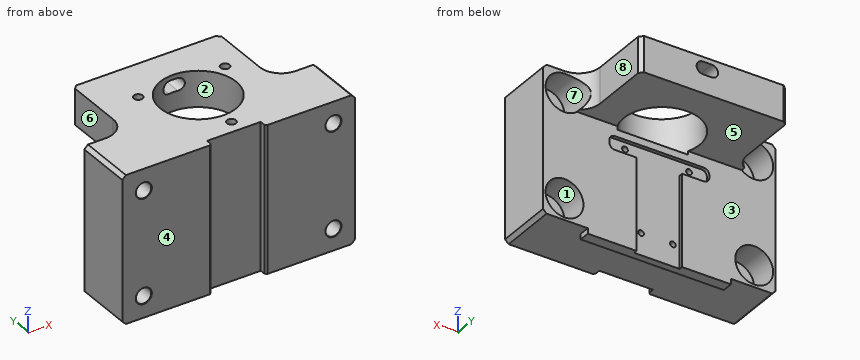
from build123d import *

# Parameters (mm, degrees)
SKETCH1_W                                     = 65
SKETCH1_H                                     = 41
BOSS_EXTRUDE1_DEPTH                           = 16
SKETCH15_W                                    = 41
SKETCH15_H                                    = 10
BOSS_EXTRUDE4_DEPTH                           = 23
SKETCH4_R                                     = 10.6
CUT_EXTRUDE3_DEPTH                            = 11
M3_TAPPED_HOLE1_D                             = 2.5
M3_TAPPED_HOLE1_DEPTH                         = 8.5
M3_TAPPED_HOLE1_TIP                           = 0.751075774
CUT_EXTRUDE4_START                            = -1
CUT_EXTRUDE4_DEPTH                            = 1
SKETCH30_W                                    = 40
SKETCH30_H                                    = 3
BOSS_EXTRUDE5_DEPTH                           = 1.5
SKETCH27_W                                    = 12.7
SKETCH27_H                                    = 4.1
CUT_EXTRUDE6_DEPTH                            = 1
CUT_EXTRUDE7_DEPTH                            = 1
M2_TAPPED_HOLE1_D                             = 1.6
M2_TAPPED_HOLE1_DEPTH                         = 6
M2_TAPPED_HOLE1_TIP                           = 0.480688495
CBORE_FOR_M4_HEX_HEAD_MACHINE_SCREW1_AT_COUNT = 2
CBORE_FOR_M4_HEX_HEAD_MACHINE_SCREW1_AT_PITCH = 53
CBORE_FOR_M4_HEX_HEAD_MACHINE_SCREW1_2_COUNT  = 2
CBORE_FOR_M4_HEX_HEAD_MACHINE_SCREW1_2_PITCH  = 60.415229868
CBORE_FOR_M4_HEX_HEAD_MACHINE_SCREW1_3_COUNT  = 2
CBORE_FOR_M4_HEX_HEAD_MACHINE_SCREW1_3_PITCH  = 29
CHAMFER4_SIZE                                 = 1
F_3_5_START                                   = 44
F_3_5_3_5_DIAMETER_SLOT1_DEPTH                = 10
FILLET1_R                                     = 6
SKETCH33_W                                    = 15
SKETCH33_H                                    = 41
CUT_EXTRUDE8_DEPTH                            = 2
CHAMFER5_SIZE                                 = 0.5


with BuildPart() as part:
    # Sketch1 → Boss-Extrude1 (new body)
    with BuildSketch(Plane(origin=(0, 15, 0), x_dir=(1, 0, 0), z_dir=(0, 1, 0))):
        with Locations((0, 20)):
            Rectangle(SKETCH1_W, SKETCH1_H)
    extrude(amount=BOSS_EXTRUDE1_DEPTH)

    # Sketch15 → Boss-Extrude4 (add)
    with BuildSketch(Plane(origin=(0, 31, 0), x_dir=(1, 0, 0), z_dir=(0, 1, 0))):
        with Locations((0, 4.5)):
            Rectangle(SKETCH15_W, SKETCH15_H)
    extrude(amount=BOSS_EXTRUDE4_DEPTH)

    # Sketch4 → Cut-Extrude3 (cut)
    with BuildSketch(Plane.XY.offset(0.5)):
        with Locations((1.85, 34.8)):
            Circle(SKETCH4_R)
    extrude(amount=-CUT_EXTRUDE3_DEPTH, mode=Mode.SUBTRACT)

    # M3 Tapped Hole1
    with Locations(Plane.XY.offset(0.5)):
        with Locations((13.974355653, 41.8), (1.85, 20.8), (-10.274355653, 41.8)):
            Hole(M3_TAPPED_HOLE1_D / 2, depth=M3_TAPPED_HOLE1_DEPTH)
            with Locations((0, 0, -(M3_TAPPED_HOLE1_DEPTH + M3_TAPPED_HOLE1_TIP / 2))):  # 118° drill point
                Cone(0, M3_TAPPED_HOLE1_D / 2, M3_TAPPED_HOLE1_TIP, mode=Mode.SUBTRACT)

    # Sketch16 → Cut-Extrude4 (cut)
    with BuildSketch(Plane(origin=(0, 31, 0), x_dir=(1, 0, 0), z_dir=(0, 1, 0)).offset(CUT_EXTRUDE4_START)):
        Polygon((-10.95, 12.5), (10.95, 12.5), (10.95, 16.3), (6.35, 16.3), (6.35, 37.9), (-6.35, 37.9), (-6.35, 16.3), (-10.95, 16.3), align=None)
    extrude(amount=CUT_EXTRUDE4_DEPTH, mode=Mode.SUBTRACT)

    # Sketch30 → Boss-Extrude5 (add)
    with BuildSketch(Plane(origin=(0, 0, -40.5), x_dir=(-1, 0, 0), z_dir=(0, 0, -1))):
        with Locations((0, 29.5)):
            Rectangle(SKETCH30_W, SKETCH30_H)
    extrude(amount=BOSS_EXTRUDE5_DEPTH)

    # Sketch27 → Cut-Extrude6 (cut)
    with BuildSketch(Plane(origin=(0, 30, 0), x_dir=(1, 0, 0), z_dir=(0, 1, 0))):
        with Locations((0, 39.95)):
            Rectangle(SKETCH27_W, SKETCH27_H)
    extrude(amount=CUT_EXTRUDE6_DEPTH, mode=Mode.SUBTRACT)

    # Sketch28 → Cut-Extrude7 (cut)
    with BuildSketch(Plane(origin=(0, 30, 0), x_dir=(1, 0, 0), z_dir=(0, 1, 0))):
        with BuildLine():
            Line((10.95, 12.5), (12.45, 12.5))
            ThreePointArc((12.45, 12.5), (13.510660172, 12.939339828), (13.95, 14))
            Line((13.95, 14), (13.95, 14.8))
            ThreePointArc((13.95, 14.8), (13.510660172, 15.860660172), (12.45, 16.3))
            Line((12.45, 16.3), (10.95, 16.3))
            Line((10.95, 16.3), (10.95, 12.5))
        make_face()
    cut_extrude7 = extrude(amount=CUT_EXTRUDE7_DEPTH, mode=Mode.SUBTRACT)

    # Mirror1: Cut-Extrude7 across plane
    add(cut_extrude7.mirror(Plane(origin=(0, 0, 0), x_dir=(0, 0, 1), z_dir=(1, 0, 0))), mode=Mode.SUBTRACT)

    # M2 Tapped Hole1
    with Locations(Plane(origin=(0, 30, 0), x_dir=(1, 0, 0), z_dir=(0, 1, 0))):
        with Locations((-4.45, 35.9), (4.45, 35.9), (8.95, 14.4), (-8.95, 14.4)):
            Hole(M2_TAPPED_HOLE1_D / 2, depth=M2_TAPPED_HOLE1_DEPTH)
            with Locations((0, 0, -(M2_TAPPED_HOLE1_DEPTH + M2_TAPPED_HOLE1_TIP / 2))):  # 118° drill point
                Cone(0, M2_TAPPED_HOLE1_D / 2, M2_TAPPED_HOLE1_TIP, mode=Mode.SUBTRACT)

    # Sketch21 → CBORE for M4 Hex Head Machine Screw1 (revolve, cut)
    with BuildSketch(Plane(origin=(26.5, 31, -34.5), x_dir=(0, 0, 1), z_dir=(1, 0, 0))):
        Polygon((0, 0), (0, 16), (2.25, 16), (2.15, 15.9), (2.15, 8), (5.295, 8), (5.295, 0), align=None)
    cbore_for_m4_hex_head_machine_screw1 = revolve(axis=Axis((26.5, 37.35, -34.5), (0, -1, 0)), mode=Mode.SUBTRACT)

    # CBORE for M4 Hex Head Machine Screw1 at: CBORE for M4 Hex Head Machine Screw1 ×2
    with Locations(*[(-i * CBORE_FOR_M4_HEX_HEAD_MACHINE_SCREW1_AT_PITCH, 0, 0) for i in range(1, CBORE_FOR_M4_HEX_HEAD_MACHINE_SCREW1_AT_COUNT)]):
        add(cbore_for_m4_hex_head_machine_screw1, mode=Mode.SUBTRACT)

    # CBORE for M4 Hex Head Machine Screw1 2: CBORE for M4 Hex Head Machine Screw1 ×2
    with Locations(*[Vector(-0.8772622419185101, 0, 0.4800114153893735) * (i * CBORE_FOR_M4_HEX_HEAD_MACHINE_SCREW1_2_PITCH) for i in range(1, CBORE_FOR_M4_HEX_HEAD_MACHINE_SCREW1_2_COUNT)]):
        add(cbore_for_m4_hex_head_machine_screw1, mode=Mode.SUBTRACT)

    # CBORE for M4 Hex Head Machine Screw1 3: CBORE for M4 Hex Head Machine Screw1 ×2
    with Locations(*[(0, 0, i * CBORE_FOR_M4_HEX_HEAD_MACHINE_SCREW1_3_PITCH) for i in range(1, CBORE_FOR_M4_HEX_HEAD_MACHINE_SCREW1_3_COUNT)]):
        add(cbore_for_m4_hex_head_machine_screw1, mode=Mode.SUBTRACT)

    # Chamfer4
    chamfer4_edges = [part.edges().sort_by_distance(p)[0] for p in [
        (-20.5, 54, -4.5),
        (20.5, 54, -4.5),
        (32.5, 23, 0.5),
        (-32.5, 23, 0.5),
        (32.5, 23, -40.5),
        (-32.5, 23, -40.5),
    ]]
    chamfer(chamfer4_edges, length=CHAMFER4_SIZE)

    # Ø3.5 (3.5) Diameter Slot1: read off the stored shape, not the designer's step
    # Ø3.5 (3.5) Diameter Slot1 outline → Ø3.5 (3.5) Diameter Slot1 (cut)
    with BuildSketch(Plane(origin=(0, 0, 0), x_dir=(1, 0, 0), z_dir=(0, 1, 0)).offset(F_3_5_START)):
        with BuildLine():
            Line((0.6, 0.8035), (3.1, 0.8035))
            ThreePointArc((3.1, 0.8035), (4.85, 2.5535), (3.1, 4.3035))
            Line((3.1, 4.3035), (0.6, 4.3035))
            ThreePointArc((0.6, 4.3035), (-1.15, 2.5535), (0.6, 0.8035))
        make_face()
    extrude(amount=F_3_5_3_5_DIAMETER_SLOT1_DEPTH, mode=Mode.SUBTRACT)

    # Fillet1
    # the kernel refuses this fillet: 6 mm, written as the material it adds along each edge
    with BuildSketch(Plane(origin=(20.5, 31, 0.5), x_dir=(1, 0, 0), z_dir=(0, 0, -1))) as fillet1_piece_1_section:
        with BuildLine():
            CenterArc((FILLET1_R, -FILLET1_R), FILLET1_R, 90, 90)
            Line((0, -FILLET1_R), (0, 0))
            Line((0, 0), (FILLET1_R, 0))
        make_face()
    fillet1_piece_1 = extrude(amount=10, mode=Mode.PRIVATE)
    fillet1_piece_1 = fillet1_piece_1 - Plane(origin=(26.5, 31, -5.5), x_dir=(0, 0, 1), z_dir=(0, 1, 0)) * Cylinder(5.295, 45, mode=Mode.PRIVATE)
    add(fillet1_piece_1)
    with BuildSketch(Plane(origin=(-20.5, 31, -9.5), x_dir=(-1, 0, 0), z_dir=(0, 0, 1))) as fillet1_piece_2_section:
        with BuildLine():
            CenterArc((FILLET1_R, -FILLET1_R), FILLET1_R, 90, 90)
            Line((0, -FILLET1_R), (0, 0))
            Line((0, 0), (FILLET1_R, 0))
        make_face()
    fillet1_piece_2 = extrude(amount=10, mode=Mode.PRIVATE)
    fillet1_piece_2 = fillet1_piece_2 - Plane(origin=(-26.5, 31, -5.5), x_dir=(0, 0, 1), z_dir=(0, 1, 0)) * Cylinder(5.295, 45, mode=Mode.PRIVATE)
    add(fillet1_piece_2)

    # Sketch33 → Cut-Extrude8 (cut)
    with BuildSketch(Plane.XZ.offset(-15)):
        with Locations((0, -20)):
            Rectangle(SKETCH33_W, SKETCH33_H)
    extrude(amount=-CUT_EXTRUDE8_DEPTH, mode=Mode.SUBTRACT)

    # Chamfer5
    chamfer5_edges = [part.edges().sort_by_distance(p)[0] for p in [
        (7.5, 15, -20),
        (-7.5, 15, -20),
    ]]
    chamfer(chamfer5_edges, length=CHAMFER5_SIZE)


solid = part.part
For this review, take the finished solid that the model builds, in its own axes (mm). Face numbers are marked on the shaded views. A direction names the side the tool comes from. Round coordinates to 2 decimals unless told otherwise and drop trailing zeros. Loops run counter-clockwise (first coordinate to the right, second up) from the corner with the lowest first, then second, coordinate; pieces in that order, holes last. Notation, with made-up numbers: (15.25, -4.75) - (27.25, -4.75) arc R27 cw to (27.25, 22.25) - close; hole circle Ø3 at (26.25, 32.25). An arc over 180 degrees is marked (long way). One line per item, written item: value. Start each with the question number.
Item 1: The part is to be moulded in two halves that separate along Y. For the marked faces 1, 2, 3 and 4, say which applies: +Y half, -Y half, draft (parallel to the pull), parting line (faces both ways), or undercut.
Item 2: For the marked faces 5, 6, 7 and 8, list the 3-axis set-ups (+Z, -Z, +X, -X, +Y, -Y) from which the entire face can be reached by the end or side of a thin tool; tool diameter is ignored.
Item 3: For L1, parallel to X at y = 19.5, z = -5.5; L2, parallel to Z at x = -26.5, y = 17; L3, parallel to Y at x = 1.85, z = -2.5, list the stretches that pass through material, from the lowest coordinate up.
Item 4: Take a section at C-C (y = 25.5). State how many separate pieces and enclosed holes the cut face has, plus the area to 3 significant figures.
Item 5: Clearance check with flat-ended pins moving along their axes: pin 1 Ø1 at (y, z) = (49.5, -4) entering from -X; pin 2 Ø17 at (x, y) = (1.85, 34.8) entering from +Z; pin 3 Ø12 at (x, z) = (1, -24) entering from -Y. State where each tip first meets the part, or that it passes through.
Item 6: Take a section at A-A (y = 50). Give the boundary of the cut face in (x, z).
Item 7: Take a section at B-B (x = -16.5). Give the boundary of the cut face in (y, z).
Answer below:
1. face 1: draft
1. face 2: undercut
1. face 3: +Y half
1. face 4: -Y half
2. face 5: -Z, +X, -X, +Y
2. face 6: +Z, -Z, -X, +Y
2. face 7: +Y
2. face 8: +Z, -Z, +X, +Y
3. L1: x = -32.5 to -28.65, -24.35 to 24.35, 28.65 to 32.5
3. L2: z = -40.5 to -36.65, -32.35 to -7.65, -3.35 to 0.5
3. L3: y = 17 to 19.55, 22.05 to 24.2
4. separate pieces: 1
4. enclosed holes: 8
4. area: 2,190 mm2
5. pin 1: stops at x = -20.5
5. pin 2: stops at z = -10.5
5. pin 3: stops at y = 17
6. outline: (-20.5, -9.5) - (20.5, -9.5) - (20.5, 0.5) - (-20.5, 0.5) - close; hole (0.6, -4.3) - (3.1, -4.3) arc R1.75 ccw to (3.1, -0.8) - (0.6, -0.8) arc R1.75 ccw to start
7. outline: (15, -40.5) - (28, -40.5) - (28, -42) - (31, -42) - (31, -9.5) - (54, -9.5) - (54, 0.5) - (15, 0.5) - close
